from build123d import *

# Parameters (mm, degrees)
F0_W     = 57.50962
F0_H     = 32.216034
F1_DEPTH = 25.4
F3_DEPTH = 32.217035


with BuildPart() as f1:
    # F0 (on Front) → F1 (new body)
    with BuildSketch(Plane.XZ):
        Rectangle(F0_W, F0_H)
    extrude(amount=F1_DEPTH)

    # F2 (on face) → F3 (cut, through all)
    with BuildSketch(Plane.XY.offset(16.108017)):
        with BuildLine():
            Line((-13.464067, -25.4), (13.464067, -25.4))
            ThreePointArc((13.464067, -25.4), (0, -11.935933), (-13.464067, -25.4))
        make_face()
    extrude(amount=-F3_DEPTH, mode=Mode.SUBTRACT)


solid = f1.part
Input: part model. Units: mm. Frame: model coordinates. Give positions to 0.01 mm unless a question says otherwise; leave off trailing zeros. Write each loop counter-clockwise with the first axis right and the second up, starting at its lowest first coordinate (ties: lowest second). Pieces come first, ordered by that corner, then holes. Notation, with made-up numbers: M 89.25,-33.5 L 126.25,-33.5 A25 ccw 126.25,-19.5 Z; hole C 74,35.5 d2. An arc over 180 degrees is marked long. Use one line per item in the form item = value.
1. Cut plane D-D on x = 9.5. Return loops of the section in (y, z).
Outcome:
outline = M -15.86,-16.11 L 0,-16.11 L 0,16.11 L -15.86,16.11 Z
2. Cut plane A-A on y = -21.75. Return loops of the section in (x, z), and give its area (3 significant figures).
Outcome:
outline = M -28.75,-16.11 L -12.96,-16.11 L -12.96,16.11 L -28.75,16.11 Z; M 12.96,-16.11 L 28.75,-16.11 L 28.75,16.11 L 12.96,16.11 Z
area = 1,020 mm²
3. Cut plane B-B on z = -9.5. Return loops of the section in (x, y), and give its area (3 significant figures).
Outcome:
outline = M -28.75,-25.4 L -13.46,-25.4 A13.46 cw 13.46,-25.4 L 28.75,-25.4 L 28.75,0 L -28.75,0 Z
area = 1,180 mm²
4. Ray query, L1, parallel to X at y = -13.25, z = -13; L2, parallel to X at y = -18.25, z = 14; L3, parallel to Y at x = -11.5, z = -13. Return the intervals inside material, ascending.
Outcome:
L1 = -28.75 to -5.8, 5.8 to 28.75
L2 = -28.75 to -11.41, 11.41 to 28.75
L3 = -18.4 to 0
5. Mould query, pull axis X, two halves, no side actions, for faces 1 (the face through (0.3, -11.94, 0.23)), 2 (the face through (-28.755, -13, 0)), 3 (the face through (-21, -25.4, 0)). Classes: released by +X, released by -X, zero draft, split by the parting line, or undercut.
Outcome:
face_1 = undercut
face_2 = released by -X
face_3 = zero draft
6. Cut plane C-C on x = 0. Return loops of the section in (y, z), and give its area (3 significant figures).
Outcome:
outline = M -11.94,-16.11 L 0,-16.11 L 0,16.11 L -11.94,16.11 Z
area = 385 mm²
